Can you work these out from the drawing? Everything is in mm from the part's minimum corner. A direction names the side the tool comes from. Round coordinates to 2 decimals unless told otherwise and drop trailing zeros. Order: outer loops, then holes, each group sorted by start corner. A loop starts at its lowest first (then second) coordinate and runs counter-clockwise, first axis right, second up. Notation, with made-up numbers: M 88.5,42 L 121.5,42 A29 ccw 121.5,63 Z; hole C 1.5,-4.5 d9. An arc over 180 degrees is marked long. Write item = value, one per line. Start each with the question number.
Item 1: We'd pull the mould along Z, two halves only. Please class the marked faces 3, 4 and 5: pulls with the +Z half, pulls with the -Z half, needs draft (parallel to the pull), parting line crosses it, or undercut.
Item 2: Please list where these lines run through material, in increasing order: L1, parallel to Z at x = 13.4, y = 20; L2, parallel to Z at x = 14.65, y = 10; L3, parallel to X at y = 15, z = 1.25.
Item 3: I'm going to push flat-ended pins straight in: P1, Ø5.5, axis at y = 10, z = 5, coming from the -X side; P2, Ø6, axis at y = 12.5, z = 10, coming from the -X side; P3, Ø2, axis at y = 20, z = 15, coming from the -X side; P4, Ø0.8, axis at x = 2.5, y = 1.5, coming from the +Z side. Where does each tip first touch, or does it pass through?
Item 4: For the marked faces 1 and 2, which set-ups out of +Z, -Z, +X, -X, +Y, -Y let a thin tool reach every point of the face, with its end or its side?
Item 5: I want a section at B-B, the plane y = 10. List the corners of the cut face in (x, z) for me.
Item 6: I want a section at A-A, the plane z = 5. List the corners of the cut face in (x, y) for me.
Item 7: I want a section at D-D, the plane y = 2.5. List the corners of the cut face in (x, z) for me, plus the area to 3 significant figures.
Item 8: I want a section at C-C, the plane x = 13. List the corners of the cut face in (y, z) for me.
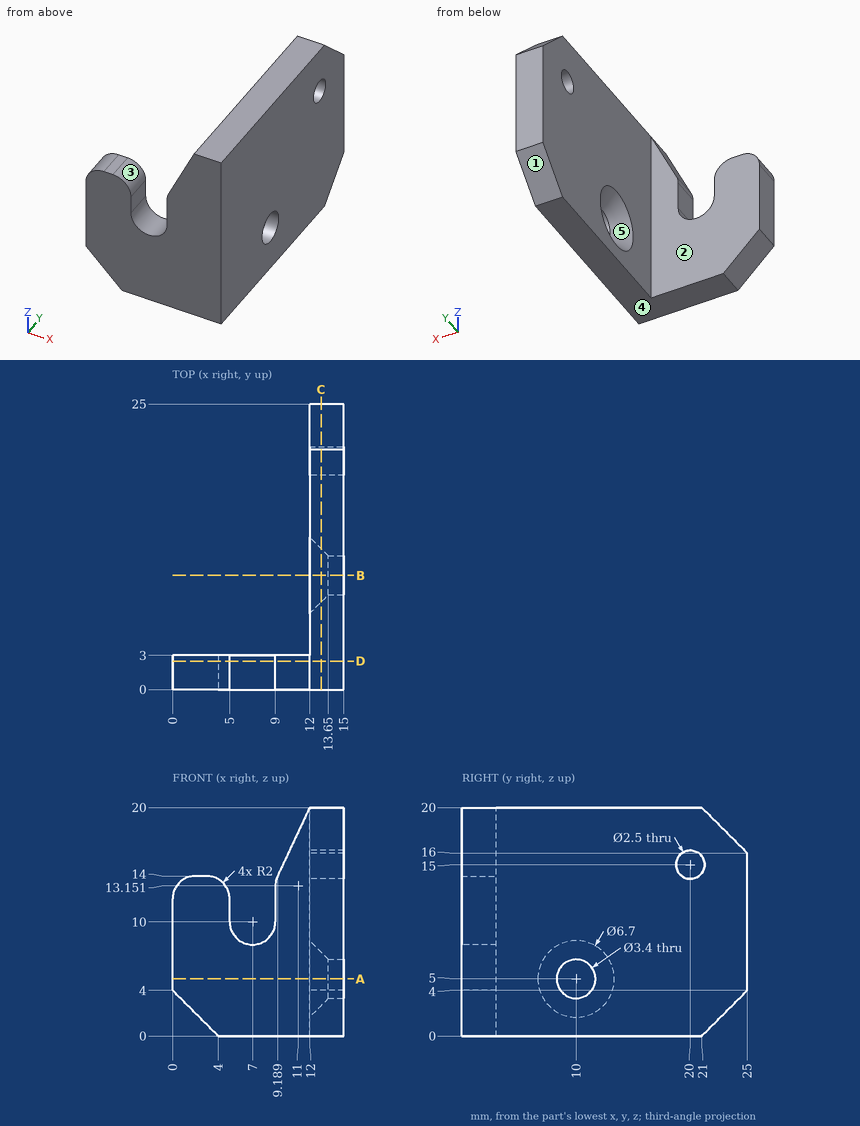
Filled in:
q1.face_3 = pulls with the +Z half
q1.face_4 = pulls with the -Z half
q1.face_5 = undercut
q2.L1 = 0 to 13.75, 16.25 to 20
q2.L2 = 0 to 3.3, 6.7 to 20
q2.L3 = 12 to 15
q3.P1 = 12.6
q3.P2 = 12
q3.P3 = through
q3.P4 = 14
q4.face_1 = -Z, +X, -X, +Y
q4.face_2 = +Z, -Z, -X, +Y
q5.outline = M 12,0 L 15,0 L 15,3.3 L 13.65,3.3 L 12,1.65 Z; M 12,8.35 L 13.65,6.7 L 15,6.7 L 15,20 L 12,20 Z
q6.outline = M 0,0 L 15,0 L 15,8.3 L 13.65,8.3 L 12,6.65 L 12,3 L 0,3 Z; M 12,13.35 L 13.65,11.7 L 15,11.7 L 15,25 L 12,25 Z
q7.outline = M 0,4 L 4,0 L 15,0 L 15,20 L 12,20 L 9.19,14 A2 ccw 9,13.15 L 9,10 A2 cw 5,10 L 5,12 A2 ccw 3,14 L 2,14 A2 ccw 0,12 Z
q7.area = 204 mm^2
q8.outline = M 0,0 L 21,0 L 25,4 L 25,16 L 21,20 L 0,20 Z; hole C 10,5 d4.7; hole C 20,15 d2.5
